```python
from build123d import *

# Parameters (mm, degrees)
ESTRUSIONE_ESTRUSIONE1_DEPTH         = 3
ESTRUSIONE_ESTRUSIONE1_DEPTH_BACK    = 3
SCHIZZO1_R                           = 140
SCHIZZO2_R                           = 62.5
TAGLIO_ESTRUSIONE1_DEPTH             = 199.080791598
SCHIZZO3_R                           = 2
ESTRUSIONE_ESTRUSIONE2_DEPTH         = 5
RIPETIZIONECIRCOLARE2_COUNT          = 4
SCHIZZO4_R                           = 2
ESTRUSIONE_ESTRUSIONE3_DEPTH         = 5
RIPETIZIONECIRCOLARE3_COUNT          = 4
ESTRUSIONE_ESTRUSIONE5_START         = -6
ESTRUSIONE_ESTRUSIONE5_DEPTH         = 35
RIPETIZIONECIRCOLARE10_COUNT         = 3
TAGLIO_ESTRUSIONE4_START             = -12.5
TAGLIO_ESTRUSIONE4_DEPTH             = 5
SCHIZZO13_R                          = 2
TAGLIO_ESTRUSIONE5_DEPTH             = 5
TAGLIO_ESTRUSIONE5_DIRECTION_2_REACH = 204.849
RIPETIZIONECIRCOLARE13_COUNT         = 3
ESTRUSIONE_ESTRUSIONE6_DEPTH         = 5
RIPETIZIONECIRCOLARE14_COUNT         = 3
SCHIZZO19_R                          = 6
TAGLIO_ESTRUSIONE6_DEPTH             = 6
FORO_PER_VITE_M3_2_D                 = 3.4
RIPETIZIONECIRCOLARE17_COUNT         = 3


with BuildPart() as part:
    # Schizzo1 → Estrusione-Estrusione1 (new, two sides: drawn at the far end of the back side and taken through both)
    with BuildSketch(Plane.XY.offset(-ESTRUSIONE_ESTRUSIONE1_DEPTH_BACK)):
        Circle(SCHIZZO1_R)
    extrude(amount=ESTRUSIONE_ESTRUSIONE1_DEPTH + ESTRUSIONE_ESTRUSIONE1_DEPTH_BACK)

    # Schizzo2 → Taglio-Estrusione1 (cut, through all)
    with BuildSketch(Plane.XY.offset(3)):
        Circle(SCHIZZO2_R)
    extrude(amount=-TAGLIO_ESTRUSIONE1_DEPTH, mode=Mode.SUBTRACT)

    # Schizzo3 → Estrusione-Estrusione2 (add)
    with BuildSketch(Plane.XY.offset(3)):
        with Locations((0, 67.5)):
            Circle(SCHIZZO3_R)
    estrusione_estrusione2 = extrude(amount=ESTRUSIONE_ESTRUSIONE2_DEPTH)

    # RipetizioneCircolare2: Estrusione-Estrusione2 ×4 about axis
    ripetizionecircolare2_axis = Axis((0, 0, 0), (0, 0, 1))
    for i in range(1, RIPETIZIONECIRCOLARE2_COUNT):
        add(estrusione_estrusione2.rotate(ripetizionecircolare2_axis, i * 360 / RIPETIZIONECIRCOLARE2_COUNT))

    # Schizzo4 → Estrusione-Estrusione3 (add)
    with BuildSketch(Plane.XY.offset(3)):
        with Locations((117.461577598, 42.752517916)):
            Circle(SCHIZZO4_R)
    estrusione_estrusione3 = extrude(amount=ESTRUSIONE_ESTRUSIONE3_DEPTH)

    # RipetizioneCircolare3: Estrusione-Estrusione3 ×4 about axis
    ripetizionecircolare3_axis = Axis((0, 0, 0), (0, 0, 1))
    for i in range(1, RIPETIZIONECIRCOLARE3_COUNT):
        add(estrusione_estrusione3.rotate(ripetizionecircolare3_axis, i * 360 / RIPETIZIONECIRCOLARE3_COUNT))

    # Schizzo6 → Estrusione-Estrusione5 (add)
    with BuildSketch(Plane.XY.offset(3).offset(ESTRUSIONE_ESTRUSIONE5_START)):
        with BuildLine():
            Line((95.45941546, 95.45941546), (98.994949366, 98.994949366))
            Line((98.994949366, 98.994949366), (102.530483272, 102.530483272))
            ThreePointArc((102.530483272, 102.530483272), (125.573683549, 72.5), (140.059244812, 37.52876154))
            Line((140.059244812, 37.52876154), (135.22961568, 36.234666314))
            Line((135.22961568, 36.234666314), (130.399986549, 34.940571089))
            ThreePointArc((130.399986549, 34.940571089), (116.913429511, 67.5), (95.45941546, 95.45941546))
        make_face()
    estrusione_estrusione5 = extrude(amount=ESTRUSIONE_ESTRUSIONE5_DEPTH)

    # RipetizioneCircolare10: Estrusione-Estrusione5 ×3 about axis
    ripetizionecircolare10_axis = Axis((0, 0, 0), (0, 0, 1))
    for i in range(1, RIPETIZIONECIRCOLARE10_COUNT):
        add(estrusione_estrusione5.rotate(ripetizionecircolare10_axis, i * 360 / RIPETIZIONECIRCOLARE10_COUNT))

    # Schizzo12 → Taglio-Estrusione4 (cut)
    with BuildSketch(Plane.XY.offset(32).offset(TAGLIO_ESTRUSIONE4_START)):
        with BuildLine():
            Line((-25, -142.828568571), (-23.275862069, -132.978322463))
            ThreePointArc((-23.275862069, -132.978322463), (0, -135), (23.275862069, -132.978322463))
            Line((23.275862069, -132.978322463), (25, -142.828568571))
            ThreePointArc((25, -142.828568571), (0, -145), (-25, -142.828568571))
        make_face()
    taglio_estrusione4 = extrude(amount=TAGLIO_ESTRUSIONE4_DEPTH, mode=Mode.SUBTRACT)

    # Schizzo13 → Taglio-Estrusione5 (cut)
    with BuildSketch(Plane.XY.offset(19.5)):
        with Locations((14.232392621, -139.274689015)):
            Circle(SCHIZZO13_R)
        with Locations((-14.232392621, -139.274689015)):
            Circle(SCHIZZO13_R)
    taglio_estrusione5 = extrude(amount=-TAGLIO_ESTRUSIONE5_DEPTH, mode=Mode.SUBTRACT)

    # Schizzo13 → Taglio-Estrusione5 direction 2 (cut, up to next)
    with BuildSketch(Plane.XY.offset(19.5), mode=Mode.PRIVATE) as taglio_estrusione5_direction_2_sk1:
        with Locations((14.232392621, -139.274689015)):
            Circle(SCHIZZO13_R)
    taglio_estrusione5_direction_2_tool1 = extrude(taglio_estrusione5_direction_2_sk1.sketch, amount=TAGLIO_ESTRUSIONE5_DIRECTION_2_REACH, mode=Mode.PRIVATE) & part.part
    # Schizzo13 → Taglio-Estrusione5 direction 2 (cut, up to next)
    with BuildSketch(Plane.XY.offset(19.5), mode=Mode.PRIVATE) as taglio_estrusione5_direction_2_sk2:
        with Locations((-14.232392621, -139.274689015)):
            Circle(SCHIZZO13_R)
    taglio_estrusione5_direction_2_tool2 = extrude(taglio_estrusione5_direction_2_sk2.sketch, amount=TAGLIO_ESTRUSIONE5_DIRECTION_2_REACH, mode=Mode.PRIVATE) & part.part
    taglio_estrusione5_direction_2_1 = taglio_estrusione5_direction_2_tool1.solids().sort_by_distance((14.232393, -139.274689, 19.5))[0]
    add(taglio_estrusione5_direction_2_1, mode=Mode.SUBTRACT)
    taglio_estrusione5_direction_2_2 = taglio_estrusione5_direction_2_tool2.solids().sort_by_distance((-14.232393, -139.274689, 19.5))[0]
    add(taglio_estrusione5_direction_2_2, mode=Mode.SUBTRACT)
    taglio_estrusione5_direction_2 = taglio_estrusione5_direction_2_1 + taglio_estrusione5_direction_2_2  # Taglio-Estrusione5 direction 2 as one shape, for the pattern or mirror that repeats it

    # RipetizioneCircolare13: Taglio-Estrusione4, Taglio-Estrusione5, Taglio-Estrusione5 direction 2 ×3 about axis
    ripetizionecircolare13_axis = Axis((0, 0, 0), (0, 0, 1))
    add([taglio_estrusione4.rotate(ripetizionecircolare13_axis, i * 360 / RIPETIZIONECIRCOLARE13_COUNT) for i in range(1, RIPETIZIONECIRCOLARE13_COUNT)], mode=Mode.SUBTRACT)
    add([taglio_estrusione5.rotate(ripetizionecircolare13_axis, i * 360 / RIPETIZIONECIRCOLARE13_COUNT) for i in range(1, RIPETIZIONECIRCOLARE13_COUNT)], mode=Mode.SUBTRACT)
    add([taglio_estrusione5_direction_2.rotate(ripetizionecircolare13_axis, i * 360 / RIPETIZIONECIRCOLARE13_COUNT) for i in range(1, RIPETIZIONECIRCOLARE13_COUNT)], mode=Mode.SUBTRACT)

    # Schizzo14 → Estrusione-Estrusione6 (add)
    with BuildSketch(Plane(origin=(0, 0, -3), x_dir=(-1, 0, 0), z_dir=(0, 0, -1))):
        with BuildLine():
            ThreePointArc((-102.636327137, 102.42453003), (-111.076444252, 93.204203405), (-118.691082442, 83.291217717))
            ThreePointArc((-118.691082442, 83.291217717), (-120.651999791, 101.239048526), (-102.636327137, 102.42453003))
        make_face()
        with BuildLine():
            ThreePointArc((-131.477851676, 61.143883739), (-148.001587774, 53.868172574), (-140.020408545, 37.673401637))
            ThreePointArc((-140.020408545, 37.673401637), (-136.255430014, 49.592920782), (-131.477851676, 61.143883739))
        make_face()
    estrusione_estrusione6 = extrude(amount=-ESTRUSIONE_ESTRUSIONE6_DEPTH)

    # RipetizioneCircolare14: Estrusione-Estrusione6 ×3 about axis
    ripetizionecircolare14_axis = Axis((0, 0, 0), (0, 0, 1))
    for i in range(1, RIPETIZIONECIRCOLARE14_COUNT):
        add(estrusione_estrusione6.rotate(ripetizionecircolare14_axis, i * 360 / RIPETIZIONECIRCOLARE14_COUNT))

    # Schizzo19 → Taglio-Estrusione6 (cut)
    with BuildSketch(Plane.XY.offset(3)):
        with Locations((-72.875773723, 12.849965147)):
            Circle(SCHIZZO19_R)
        with Locations((47.566283117, 56.687288791)):
            Circle(SCHIZZO19_R)
        with Locations((25.309490606, -69.537253938)):
            Circle(SCHIZZO19_R)
    extrude(amount=-TAGLIO_ESTRUSIONE6_DEPTH, mode=Mode.SUBTRACT)

    # Foro per Vite M3-2 (through all)
    with Locations(Plane.XY.offset(2)):
        with Locations((-26.307698917, -149.198374581), (26.307698917, -149.198374581)):
            foro_per_vite_m3_2 = Hole(FORO_PER_VITE_M3_2_D / 2)

    # RipetizioneCircolare17: Foro per Vite M3-2 ×3 about axis
    ripetizionecircolare17_axis = Axis((0, 0, 0), (0, 0, 1))
    for i in range(1, RIPETIZIONECIRCOLARE17_COUNT):
        add(foro_per_vite_m3_2.rotate(ripetizionecircolare17_axis, i * 360 / RIPETIZIONECIRCOLARE17_COUNT), mode=Mode.SUBTRACT)


solid = part.part
```
For this review, take the finished solid that the model builds, in its own axes (mm). A direction names the side the tool comes from. Round coordinates to 2 decimals unless told otherwise and drop trailing zeros. Loops run counter-clockwise (first coordinate to the right, second up) from the corner with the lowest first, then second, coordinate; pieces in that order, holes last.
Q1. Mouldability with a two-part tool opening along Z and no side actions: class faces 4 (the face through (-135.162, 36.217, 14.255)), 5 (the face through (-120, 69, 19.5)), 6 (the face through (-120, 69, 24.5)), 7 (the face through (-64, 4, 3)) as +Z half, -Z half, draft (parallel to the pull), parting line (faces both ways), or undercut.
Result sheet:
face 4: draft
face 5: undercut
face 6: undercut
face 7: +Z half
Q2. Insertion check: pin 1 Ø4.5 at (x, y) = (-67, -0.5) entering from +Z; pin 2 Ø12 at (x, y) = (68, 33) entering from +Z; pin 3 Ø8 at (x, z) = (-2, 16) entering from -Y; pin 4 Ø11 at (x, y) = (25.31, -69.54) entering from -Z. Each pin has a flat end and moves straight along its axis. Give the tip position at first contact, or say it passes through.
Result sheet:
pin 1: stops at z = 8
pin 2: stops at z = 3
pin 3: stops at y = -145
pin 4: passes through
Q3. Machinability: for faces 1 (the face through (-113, 96, 2)), 2 (the face through (99, 99, 14)), 3 (the face through (140, 50, 2)), which of the approach directions +Z, -Z, +X, -X, +Y, -Y give a long, thin tool a straight path to every point of the face, cutting with its end or side? Answer none if there is none.
Result sheet:
face 1: +Z, -X, +Y
face 2: +Z, +Y
face 3: +Z, +X, +Y
Q4. Add section A-A on y = -123. Write out the cut boundary in (x, z).
Result sheet:
outline: (-66.87, -3) - (66.87, -3) - (66.87, 3) - (-66.87, 3) - close
Q5. To check wall thickness, follow line 1 along Z through (x, y) = (-94, 37); line 2 along Y through (x, z) = (-114, 16); line 3 along X through (y, z) = (74, 29). State the ranges of each line that lie inside material, in increasing order.
Result sheet:
line 1: z = -3 to 3
line 2: y = 72.31 to 80.03, 83.9 to 89.6
line 3: x = -124.7 to -112.91, 112.91 to 124.7
